Read the model definition and answer for the solid it produces. Units are mm, in the model's axes. A direction names the side the tool comes from. Round coordinates to 2 decimals unless told otherwise and drop trailing zeros. Order: outer loops, then holes, each group sorted by start corner. A loop starts at its lowest first (then second) coordinate and runs counter-clockwise, first axis right, second up. Notation, with made-up numbers: (19.5, 67) - (27.5, 67) arc R32 cw to (27.5, 103) - close; hole circle Ø10 at (32, 52.5). An arc over 180 degrees is marked (long way). One line per question, with ' | ' between items. Start each with the question number.
1) The part is cut by section B-B, the plane y = 2.13. Give the vertices of the cut face in (x, z), plus the area to 3 significant figures.
2) The part is cut by section C-C, the plane x = 2.5. Give the vertices of the cut face in (y, z).
3) The mould has two halves that part along X. Classify faces 1 (the flat face through (18, 13, 2)), 2 (the flat face through (8, 19.05, 1)), 3 (the flat face through (39, 12, 1)): pulls with the +X half, pulls with the -X half, needs draft (parallel to the pull), parting line crosses it, or undercut.
4) A flat-ended cylindrical pin translates along its axis: pin 1 (1.8 mm diameter, centred on x = 2.13, y = 22.97, fed in from +Z). Find the tip coordinate at first contact, or state that the pin passes through.
5) The part is cut by section D-D, the plane z = 1.65. Give the vertices of the cut face in (x, y), plus the area to 3 significant figures.
6) Straight lines are drawn through the part: line 1 (Y direction, x = 2.13, z = 0.95); line 2 (X direction, y = 2.13, z = 1.3); line 3 (X direction, y = 10.75, z = 1.4). For each, find the intervals that lie inside material, in ascending order. Write a range as from..to.
7) For faces 4 (the flat face through (18, 13, 0)), 5 (the flat face through (1.597, 13, 1)), determine the directions among +Z, -Z, +X, -X, +Y, -Y from which every point of the face is accessible in a straight line to the end or side of a thin tool.
8) The part is cut by section A-A, the plane x = 8. Give the vertices of the cut face in (y, z).
from build123d import *

# Parameters (mm, degrees)
ESBO_O1_W                = 35
ESBO_O1_H                = 25.1
RESSALTO_EXTRUS_O1_DEPTH = 2
ESBO_O2_R                = 1.5
CORTE_EXTRUS_O1_DEPTH    = 2
ESBO_O3_W                = 2.002857319
ESBO_O3_H                = 25.1
RESSALTO_EXTRUS_O2_DEPTH = 2
CORTE_EXTRUS_O2_DEPTH    = 2
ESBO_O5_W                = 4
ESBO_O5_H                = 25.1
RESSALTO_EXTRUS_O3_DEPTH = 2


with BuildPart() as part:
    # Esboço1 → Ressalto-extrusão1 (new body)
    with BuildSketch(Plane.XY):
        with Locations((17.5, 12.55)):
            Rectangle(ESBO_O1_W, ESBO_O1_H)
    extrude(amount=RESSALTO_EXTRUS_O1_DEPTH)

    # Esboço2 → Corte-extrusão1 (cut)
    with BuildSketch(Plane.XY.offset(2)):
        with Locations((2.13, 22.97)):
            Circle(ESBO_O2_R)
        with Locations(Location((2.13, 2.13, 0), (0, 0, 180))):
            Circle(ESBO_O2_R)
    extrude(amount=-CORTE_EXTRUS_O1_DEPTH, mode=Mode.SUBTRACT)

    # Esboço3 → Ressalto-extrusão2 (add)
    with BuildSketch(Plane.XY.offset(2)):
        with Locations((-1.00142866, 12.55)):
            Rectangle(ESBO_O3_W, ESBO_O3_H)
    extrude(amount=-RESSALTO_EXTRUS_O2_DEPTH)

    # Esboço4 → Corte-extrusão2 (cut)
    with BuildSketch(Plane.XY.offset(2)):
        Polygon((1.597142681, 12.55), (1.597142681, 19.05), (14.597142681, 19.05), (14.597142681, 6.05), (1.597142681, 6.05), align=None)
    extrude(amount=-CORTE_EXTRUS_O2_DEPTH, mode=Mode.SUBTRACT)

    # Esboço5 → Ressalto-extrusão3 (add)
    with BuildSketch(Plane.XY.offset(2)):
        with Locations((37, 12.55)):
            Rectangle(ESBO_O5_W, ESBO_O5_H)
    extrude(amount=-RESSALTO_EXTRUS_O3_DEPTH)


solid = part.part
Values:
1) outline: (-2, 0) - (0.63, 0) - (0.63, 2) - (-2, 2) - close; (3.63, 0) - (39, 0) - (39, 2) - (3.63, 2) - close | area: 76.0 mm^2
2) outline: (0, 0) - (0.68, 0) - (0.68, 2) - (0, 2) - close; (3.58, 0) - (6.05, 0) - (6.05, 2) - (3.58, 2) - close; (19.05, 0) - (21.52, 0) - (21.52, 2) - (19.05, 2) - close; (24.42, 0) - (25.1, 0) - (25.1, 2) - (24.42, 2) - close
3) face 1: needs draft | face 2: undercut | face 3: pulls with the +X half
4) pin 1: passes through
5) outline: (-2, 0) - (39, 0) - (39, 25.1) - (-2, 25.1) - close; hole circle Ø3 at (2.13, 2.13); hole circle Ø3 at (2.13, 22.97); hole (1.6, 6.05) - (14.6, 6.05) - (14.6, 19.05) - (1.6, 19.05) - close | area: 846 mm^2
6) line 1: y = 0..0.63, 3.63..6.05, 19.05..21.47, 24.47..25.1 | line 2: x = -2..0.63, 3.63..39 | line 3: x = -2..1.6, 14.6..39
7) face 4: -Z, +X, -X, +Y, -Y | face 5: +Z, -Z
8) outline: (0, 0) - (6.05, 0) - (6.05, 2) - (0, 2) - close; (19.05, 0) - (25.1, 0) - (25.1, 2) - (19.05, 2) - close
